Check sheet for the modelled part. Datum: model origin and axes. Units: mm. Face numbers are marked on the shaded views. A direction names the side the tool comes from. Round coordinates to 2 decimals unless told otherwise and drop trailing zeros. Write each loop counter-clockwise with the first axis right and the second up, starting at its lowest first coordinate (ties: lowest second). Pieces come first, ordered by that corner, then holes. Notation, with made-up numbers: (14.5, 20.25) -> (25.5, 20.25) arc R31 cw to (25.5, 51.25) -> close; hole circle Ø4 at (76.25, 19). An arc over 180 degrees is marked (long way). One line per item, written item: value.
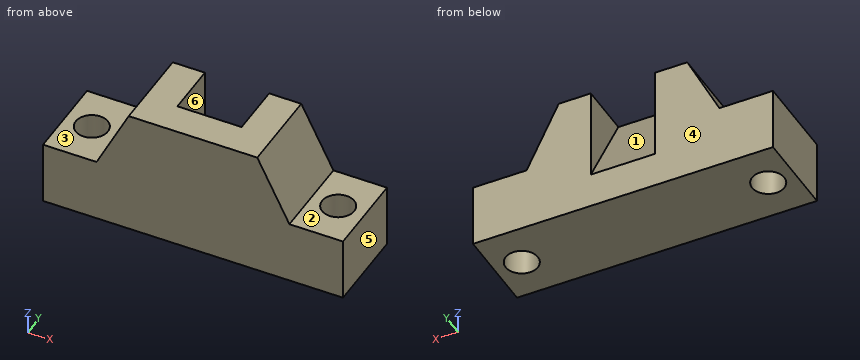
from build123d import *

# Parameters (mm, degrees)
F1_DEPTH    = 40
F2_W        = 30
F2_H        = 45
F3_DEPTH    = 25
F4_T4_DEPTH = 30
F5_R        = 7.5
F6_DEPTH    = 30


# Not quite as in the source:
# - a fillet or chamfer that OpenCascade refuses, or shapes differently, is made with other operations: its cross-section is extruded or revolved along the edge and cut away or added


with BuildPart() as f1:
    # F0 (on Front) → F1 (new body)
    with BuildSketch(Plane.XZ):
        Polygon((0, 30), (0, 0), (140, 0), (140, 30), (115, 30), (100, 60), (85, 60), (55, 60), (40, 60), (25, 30), align=None)
    extrude(amount=F1_DEPTH)

    # F2 (on Front) → F3 (cut)
    with BuildSketch(Plane.XZ):
        with Locations((70, 37.5)):
            Rectangle(F2_W, F2_H)
    extrude(amount=F3_DEPTH, mode=Mode.SUBTRACT)

    # F4: chamfer of 45 x 25.9807621135 on 1 edges, made by hand


with BuildPart() as f4_tool2:
    # F4_s3 → F4_t4 (new body)
    with BuildSketch(Plane.YZ.offset(55)):
        Polygon((0.9807621135, 15), (-25, 60), (-25, 15), align=None)
    extrude(amount=F4_T4_DEPTH)

    split(bisect_by=Plane.XZ, keep=Keep.TOP)

    split(bisect_by=Plane.XY.offset(60), keep=Keep.BOTTOM)


with BuildPart() as f1_1:
    add(f1.part)

    # F4_t1: union F4_tool2
    add(f4_tool2.part)

    # F5 (on Top) → F6 (cut)
    with BuildSketch(Plane.XY):
        with Locations((127.5, -20)):
            Circle(F5_R)
        with BuildLine():
            ThreePointArc((12.5, -12.5), (7.1966991411, -25.3033008589), (20, -20))
            ThreePointArc((20, -20), (17.8033008589, -14.6966991411), (12.5, -12.5))
        make_face()
    extrude(amount=F6_DEPTH, mode=Mode.SUBTRACT)


solid = f1_1.part
Item 1: Sectioned sample at B-B (y = -20). Enter the section's corners in (x, z), then the cut area to 3 significant figures.
Result set:
outline: (0, 0) -> (5, 0) -> (5, 30) -> (0, 30) -> close; (20, 0) -> (120, 0) -> (120, 30) -> (115, 30) -> (100, 60) -> (85, 60) -> (85, 51.34) -> (55, 51.34) -> (55, 60) -> (40, 60) -> (25, 30) -> (20, 30) -> close; (135, 0) -> (140, 0) -> (140, 30) -> (135, 30) -> close
area: 5,290 mm^2
Item 2: Sectioned sample at D-D (z = 19). Enter the section's corners in (x, y), then the cut area to 3 significant figures.
Result set:
outline: (0, -40) -> (140, -40) -> (140, 0) -> (85, 0) -> (85, -1.33) -> (55, -1.33) -> (55, 0) -> (0, 0) -> close; hole circle Ø15 at (12.5, -20); hole circle Ø15 at (127.5, -20)
area: 5,210 mm^2
Item 3: Depth check by flat-ended pin: pin 1 (20 mm diameter, centred on x = 127.5, y = -18.5, fed in from +Z); pin 2 (7.5 mm diameter, centred on y = -13.5, z = 38.5, fed in from +X) (3 decimals); pin 3 (1 mm diameter, centred on x = 122.5, z = 32, fed in from +Y); pin 4 (1 mm diameter, centred on x = 111, y = -27, fed in from +Z). Enter the tip coordinate at first touch or a pass-through.
Result set:
pin 1: z = 30
pin 2: x = 112.625
pin 3: through
pin 4: z = 39
Item 4: Material ranges on line 1 along Y through (x, z) = (127, 12); line 2 along X through (y, z) = (-15, 19.5); line 3 along X through (y, z) = (-19, 18.5), recorded low to high.
Result set:
line 1: -40 to -27.48, -12.52 to 0
line 2: 0 to 6.91, 18.09 to 121.91, 133.09 to 140
line 3: 0 to 5.07, 19.93 to 120.07, 134.93 to 140
Item 5: Tool access check on the marked faces 1, 2 and 3. Record the directions out of +Z, -Z, +X, -X, +Y, -Y that give a thin tool (end or side, any length) a straight path to the whole face; none if there is none.
Result set:
face 1: +Z, +Y
face 2: +Z, +X, +Y, -Y
face 3: +Z, -X, +Y, -Y
Item 6: Sectioned sample at A-A (x = 127.5). Enter the section's corners in (y, z), then the cut area to 3 significant figures.
Result set:
outline: (-40, 0) -> (-27.5, 0) -> (-27.5, 30) -> (-40, 30) -> close; (-12.5, 0) -> (0, 0) -> (0, 30) -> (-12.5, 30) -> close
area: 750 mm^2
Item 7: Sectioned sample at C-C (y = -34). Enter the section's corners in (x, z).
Result set:
outline: (0, 0) -> (140, 0) -> (140, 30) -> (115, 30) -> (100, 60) -> (40, 60) -> (25, 30) -> (0, 30) -> close
Item 8: Release check for a two-part mould opening along X. For the marked faces 4, 5 and 6 record: pulls with the +X half, pulls with the -X half, needs draft (parallel to the pull), parting line crosses it, or undercut.
Result set:
face 4: needs draft
face 5: pulls with the +X half
face 6: undercut
